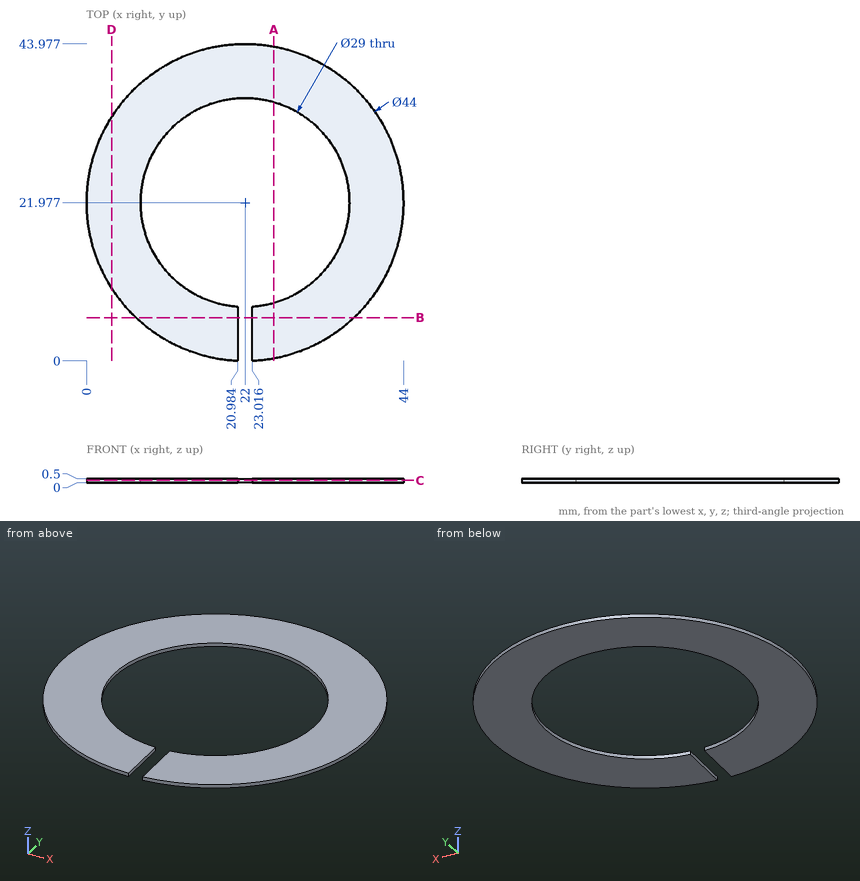
For this review, use the dimensioned drawing (mm, ordinates from the lowest corner) and the shaded views. Round coordinates to 2 decimals unless told otherwise and drop trailing zeros. Order: outer loops, then holes, each group sorted by start corner. A loop starts at its lowest first (then second) coordinate and runs counter-clockwise, first axis right, second up. Notation, with made-up numbers: (79, 11) -> (91, 11) arc R23 cw to (91, 38) -> close; hole circle Ø3 at (68, 40.25). An arc over 180 degrees is marked (long way). Write item = value, one per line. Start each with the question number.
Item 1: For line 1 along Y through (x, z) = (22, 0.25); line 2 along X through (y, z) = (12.5, 0.4) (1 decimal); line 3 along X through (y, z) = (22.5, 0.2), list the stretches that pass through material, from the lowest coordinate up.
Item 2: Consider section A-A on x = 26. Write out the cut boundary in (y, z).
Item 3: Consider section B-B on y = 6. Write out the cut boundary in (x, z) (1 decimal).
Item 4: Consider section D-D on x = 3.5. Write out the cut boundary in (y, z).
Item 5: Consider section C-C on z = 0.3. Write out the cut boundary in (x, y) (1 decimal).
Conclusion:
q1.line_1 = 36.48 to 43.98
q1.line_2 = 2.1 to 11, 33 to 41.9
q1.line_3 = 0.01 to 7.51, 36.49 to 43.99
q2.outline = (0.34, 0) -> (8.04, 0) -> (8.04, 0.5) -> (0.34, 0.5) -> close; (35.91, 0) -> (43.61, 0) -> (43.61, 0.5) -> (35.91, 0.5) -> close
q3.outline = (6.9, 0) -> (21, 0) -> (21, 0.5) -> (6.9, 0.5) -> close; (23, 0) -> (37.1, 0) -> (37.1, 0.5) -> (23, 0.5) -> close
q4.outline = (10.07, 0) -> (33.88, 0) -> (33.88, 0.5) -> (10.07, 0.5) -> close
q5.outline = (21, 0) -> (21, 7.5) arc R14.5 cw (long way) to (23, 7.5) -> (23, 0) arc R22 ccw (long way) to start
